```python
from build123d import *

# Parameters (mm, degrees)
F0_W     = 50
F0_H     = 5
F1_DEPTH = 5
F2_D     = 3.5
F3_R     = 3
F5_D     = 2.95


with BuildPart() as f1:
    # F0 (on Front) → F1 (new body)
    with BuildSketch(Plane.XZ):
        Rectangle(F0_W, F0_H)
    extrude(amount=-F1_DEPTH)

    # F2 (through all)
    with Locations(Plane.XZ):
        with Locations((-10, 0), (10, 0)):
            Hole(F2_D / 2)

    # F3
    f3_edges = [f1.edges().sort_by_distance(p)[0] for p in [
        (-25, 0, 0),
        (25, 0, 0),
    ]]
    fillet(f3_edges, radius=F3_R)

    # F5 (through all)
    with Locations(Plane.XY.offset(2.5)):
        with Locations((-20, 5), (0, 5), (20, 5)):
            Hole(F5_D / 2)


solid = f1.part
```
Check sheet for the modelled part. Datum: model origin and axes. Units: mm. Give positions to 0.01 mm unless a question says otherwise; leave off trailing zeros. Loops run counter-clockwise (first coordinate to the right, second up) from the corner with the lowest first, then second, coordinate; pieces in that order, holes last. Notation, with made-up numbers: (9, -16.5) - (51, -16.5) arc R24 ccw to (51, 8.5) - close; hole circle Ø10 at (78, 81). An arc over 180 degrees is marked (long way). One line per question, with ' | ' between items. Start each with the question number.
1. Cross-section at D-D, the plane x = -20. Enter the section's corners in (y, z) (3 decimals), plus the area to 3 significant figures.
2. Cross-section at C-C, the plane y = 1.05. Enter the section's corners in (x, z), plus the area to 3 significant figures.
3. Gauge pin test, flat end, axial feed: pin 1 Ø3 at (y, z) = (0.5, -1.5) entering from +X. Record the tip position at first contact, or that the pin passes through.
4. Material ranges on line 1 along X through (y, z) = (1.95, -0.9); line 2 along X through (y, z) = (3.9, -1.05); line 3 along X through (y, z) = (4.75, -1.95), recorded low to high. Write a range as [from, to].
5. Cross-section at B-B, the plane x = -10. Enter the section's corners in (y, z).
6. Cross-section at A-A, the plane z = 0. Enter the section's corners in (x, y) (3 decimals), plus the area to 3 significant figures.
Check result:
1) outline: (0, -2.5) - (3.525, -2.5) - (3.525, 2.5) - (0, 2.5) - close | area: 17.6 mm2
2) outline: (-24.28, -2.5) - (24.28, -2.5) - (24.28, 2.5) - (-24.28, 2.5) - close; hole circle Ø3.5 at (-10, 0); hole circle Ø3.5 at (10, 0) | area: 224 mm2
3) pin 1: stops at x = 24.83
4) line 1: x = [-24.81, -11.5], [-8.5, 8.5], [11.5, 24.81] | line 2: x = [-25, -20.98], [-19.02, -11.4], [-8.6, -0.98], [0.98, 8.6], [11.4, 19.02], [20.98, 25] | line 3: x = [-25, -21.45], [-18.55, -1.45], [1.45, 18.55], [21.45, 25]
5) outline: (0, -2.5) - (5, -2.5) - (5, -1.75) - (0, -1.75) - close; (0, 1.75) - (5, 1.75) - (5, 2.5) - (0, 2.5) - close
6) outline: (-25, 3) arc R3 ccw to (-22, 0) - (-11.75, 0) - (-11.75, 5) - (-18.525, 5) arc R1.475 cw to (-21.475, 5) - (-25, 5) - close; (-8.25, 0) - (8.25, 0) - (8.25, 5) - (1.475, 5) arc R1.475 cw to (-1.475, 5) - (-8.25, 5) - close; (11.75, 0) - (22, 0) arc R3 ccw to (25, 3) - (25, 5) - (21.475, 5) arc R1.475 cw to (18.525, 5) - (11.75, 5) - close | area: 201 mm2
